Here's the drawing with two shaded views (mm, measured from the low corner). I have some questions. Give positions to 0.01 mm unless a question says otherwise; leave off trailing zeros. Order: outer loops, then holes, each group sorted by start corner. A loop starts at its lowest first (then second) coordinate and runs counter-clockwise, first axis right, second up. Notation, with made-up numbers: M -20,5 L 35,5 A27 cw 35,36 Z; hole C 15,-6 d3. An arc over 180 degrees is marked long. Write each question's results on one line, items separated by ' | '.
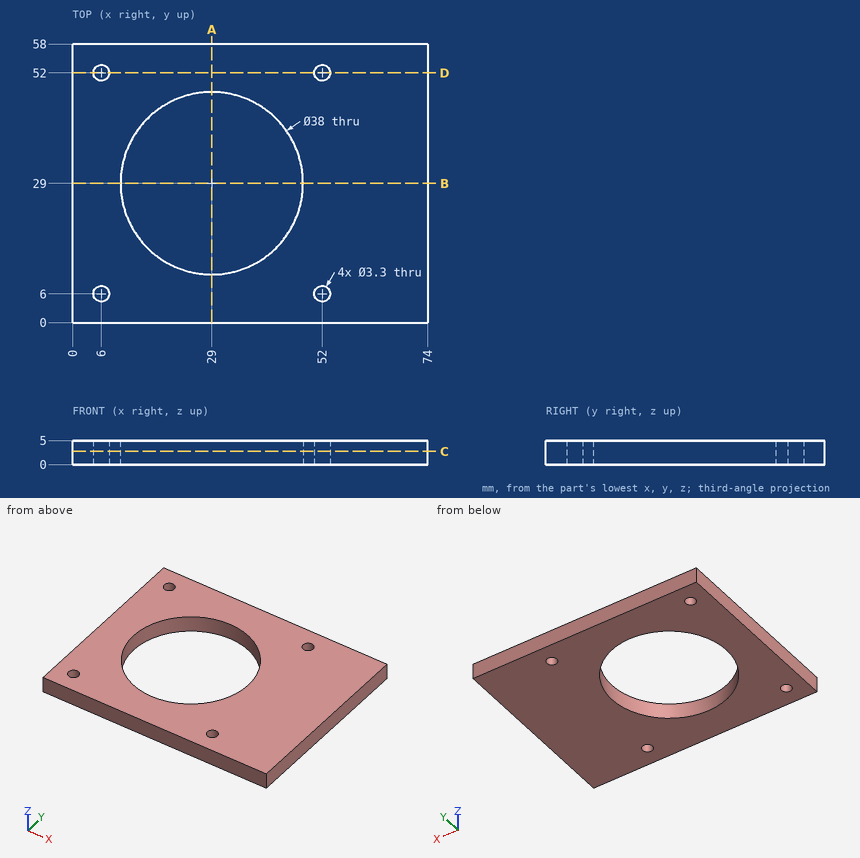
(1) Imagine slicing it at C-C, the plane z = 2.75. Write out the boundary of the cut face in (x, y).
Data:
outline: M 0,0 L 74,0 L 74,58 L 0,58 Z; hole C 6,6 d3.3; hole C 6,52 d3.3; hole C 29,29 d38; hole C 52,6 d3.3; hole C 52,52 d3.3
(2) Imagine slicing it at D-D, the plane y = 52. Write out the boundary of the cut face in (x, z), plus the area to 3 significant figures.
Data:
outline: M 0,0 L 4.35,0 L 4.35,5 L 0,5 Z; M 7.65,0 L 50.35,0 L 50.35,5 L 7.65,5 Z; M 53.65,0 L 74,0 L 74,5 L 53.65,5 Z | area: 337 mm2
(3) Will this pin go through, and if not, where does the flat tip stop? P1, Ø2, axis at x = 52, y = 6, coming from the +Z side.
Data:
P1: passes through
(4) Imagine slicing it at B-B, the plane y = 29. Write out the boundary of the cut face in (x, z).
Data:
outline: M 0,0 L 10,0 L 10,5 L 0,5 Z; M 48,0 L 74,0 L 74,5 L 48,5 Z
(5) Imagine slicing it at A-A, the plane x = 29. Write out the boundary of the cut face in (y, z).
Data:
outline: M 0,0 L 10,0 L 10,5 L 0,5 Z; M 48,0 L 58,0 L 58,5 L 48,5 Z
(6) I need wall thicknesses on L1, parallel to Y at x = 6, z = 1.9; L2, parallel to Y at x = 29, z = 2.2; L3, parallel to Y at x = 21, z = 0.7. Which ranges of each line are inside material? Lowest first, please. Write a range as from..to.
Data:
L1: y = 0..4.35, 7.65..50.35, 53.65..58 | L2: y = 0..10, 48..58 | L3: y = 0..11.77, 46.23..58
